Work out the finished part from the listing and answer in its coordinate system (mm). A direction names the side the tool comes from. Give positions to 0.01 mm unless a question says otherwise; leave off trailing zeros. Loops run counter-clockwise (first coordinate to the right, second up) from the corner with the lowest first, then second, coordinate; pieces in that order, holes last. Notation, with made-up numbers: (79, 24) - (83, 24) arc R31 cw to (83, 55) - close; hole circle Ø9 at (27, -24). An arc over 180 degrees is marked (long way). One line per question, with ' | ' between items. Start each with the question number.
1. Each of these flat-tipped pins is pushed along its axis until it touches: pin 1 (3 mm diameter, centred on y = -15, z = 40.5, fed in from +X); pin 2 (3 mm diameter, centred on y = 34, z = 35.5, fed in from +X); pin 3 (1.5 mm diameter, centred on x = 63, y = 30.5, fed in from +Z). Where does it stop, or does it pass through?
2. Section B-B (z = 13) is taken. Determine the outline of the cut face in (x, y).
3. Which of the six approach directions +Z, -Z, +X, -X, +Y, -Y give full straight-line access (tool end or side, diameter ignored) to faces 1 (the face through (90, -30, 45.974)), 2 (the face through (86, 1, 0))?
4. Find the intervals of material crossed by line 1 (Z direction, x = 50.5, y = -9.5); line 2 (Y direction, x = 119, z = 41.5); line 3 (X direction, y = -37, z = 28.5), in increasing order.
5. Section A-A (y = 0) is taken. Determine the outline of the cut face in (x, z).
6. Section C-C (z = 44) is taken. Determine the outline of the cut face in (x, y).
from build123d import *

# Parameters (mm, degrees)
F0_R     = 45.219595
F1_DEPTH = 45.974
F2_SIZE  = 5.08
F3_R     = 29.259427
F4_DEPTH = 25.4


with BuildPart() as f1:
    # F0 (on Top) → F1 (new body)
    with BuildSketch(Plane.XY):
        with Locations((86.820111, 0)):
            Circle(F0_R)
    extrude(amount=F1_DEPTH)

    # F2
    f2_edges = [f1.edges().sort_by_distance(p)[0] for p in [
        (41.600516, 0, 45.974),
    ]]
    chamfer(f2_edges, length=F2_SIZE)

    # F3 (on face) → F4 (join)
    with BuildSketch(Plane.XY.offset(45.974)):
        with Locations((86.820111, 0)):
            Circle(F3_R)
    extrude(amount=F4_DEPTH)


solid = f1.part
Conclusion:
1) pin 1: x = 129.98 | pin 2: x = 118.26 | pin 3: z = 45.97
2) outline: circle Ø90.44 at (86.82, 0)
3) face 1: +Z | face 2: -Z, +X, -X, +Y, -Y
4) line 1: 0 to 45.97 | line 2: -30.9 to 30.9 | line 3: 60.82 to 112.82
5) outline: (41.6, 0) - (132.04, 0) - (132.04, 40.89) - (126.96, 45.97) - (116.08, 45.97) - (116.08, 71.37) - (57.56, 71.37) - (57.56, 45.97) - (46.68, 45.97) - (41.6, 40.89) - close
6) outline: circle Ø84.23 at (86.82, 0)
